Autodesk Inventor part; units mm, degrees
ref_plane "YZ Plane" through (0, 0, 0) normal (1, 0, 0) x (0, 1, 0)
ref_plane "XZ Plane" through (0, 0, 0) normal (0, 1, 0) x (-1, 0, 0)
ref_plane "XY Plane" through (0, 0, 0) normal (0, 0, 1) x (1, 0, 0)
sketch "Sketch1" plane through (0, 0, 0) normal (0, 0, 1) x (1, 0, 0)
  line L0 (-11.8, 0) -> (-11.8, 3)
  line L1 (-11.8, 3) -> (-5.8, 3)
  line L2 (-5.8, 3) -> (-5.8, 11)
  line L3 (-5.8, 11) -> (-1.4, 11)
  line L4 (-1.4, 11) -> (-1.4, 3)
  line L5 (-1.4, 3) -> (1.4, 3)
  line L6 (1.4, 3) -> (1.4, 11)
  line L7 (1.4, 11) -> (5.8, 11)
  line L8 (5.8, 11) -> (5.8, 3)
  line L9 (5.8, 3) -> (11.8, 3)
  line L10 (11.8, 3) -> (11.8, 0)
  line L11 (11.8, 0) -> (-11.8, 0)
  point P0 (0, 0)
  dimension "d0" = 3
  dimension "d1" = 6
  dimension "d2" = 8
  dimension "d3" = 4.4
  dimension "d4" = 2.8
  dimension "d5" = 4.4
  dimension "d6" = 6
  dimension "d7" = 1.4
  dimension "d8" = 0
extrude "Extrusion1" add sketch "Sketch1" along normal blind 6.5
sketch "Sketch2" plane through (-11.8, 0, 0) normal (0, -1, 0) x (1, 0, 0)
  circle A0 centre (2.8, 3.25) radius 1.5
  circle A1 centre (20.8, 3.25) radius 1.5
  line L0 (23.6, 0) -> (23.6, 6.5)
  line L1 (0, 0) -> (0, 6.5)
  line L2 (23.6, 0) -> (0, 0)
  line L3 (0, 6.5) -> (23.6, 6.5)
  line L4 (11.8, 17.7341) -> (11.8, -9.1991) construction
  line L5 (10.4, 0) -> (10.4, 6.5) construction
  line L6 (13.2, 0) -> (13.2, 6.5) construction
  point P0 (11.8, 0)
  dimension "d11" = 3
  dimension "d12" = 3
  dimension "d13" = 18
  dimension "d14" = 23.6
  dimension "d15" = 2.8
  dimension "d16" = 6.5
  dimension "d17" = 3.25
  dimension "d18" = 3.25
  dimension "d34" = 2.8
  dimension "d35" = 1.4
extrude "Extrusion2" cut sketch "Sketch2" against normal through all contours A0 | A1
sketch "Sketch3" plane through (-11.8, 0, 0) normal (0, -1, 0) x (1, 0, 0)
  line L0 (-9.1, 8.25) -> (23.9, 8.25)
  line L1 (23.9, 8.25) -> (23.9, -1.75)
  line L2 (23.9, -1.75) -> (-9.1, -1.75)
  line L3 (-9.1, -1.75) -> (-9.1, 8.25)
  line L4 (23.6, 0) -> (23.6, 6.5)
  line L5 (23.6, 0) -> (0, 0)
  line L6 (0, 6.5) -> (23.6, 6.5)
  circle A0 centre (2.8, 3.25) radius 1.5
  circle A1 centre (20.8, 3.25) radius 1.5
  point P0 (11.8, 0)
  dimension "d21" = 10
  dimension "d22" = 33
  dimension "d23" = 0.3
  dimension "d24" = 6.5
  dimension "d25" = 1.75
extrude "Extrusion3" add sketch "Sketch3" along normal blind 2
sketch "Sketch4" plane through (-11.8, -2, 0) normal (0, -1, 0) x (1, 0, 0)
  line L0 (-8.8, 8.25) -> (-2.8, 8.25)
  line L1 (-2.8, 8.25) -> (-2.8, -1.75)
  line L2 (-2.8, -1.75) -> (-8.8, -1.75)
  line L3 (-8.8, -1.75) -> (-8.8, 8.25)
  line L4 (-9.1, -1.75) -> (23.9, -1.75)
  line L5 (-9.1, -1.75) -> (-9.1, 8.25)
  point P0 (11.8, 0)
  dimension "d28" = 10
  dimension "d29" = 6
  dimension "d30" = 0
  dimension "d31" = 0.3
extrude "Extrusion4" add sketch "Sketch4" along normal blind 10
equation "\"d15\" = -0.5 * d13 + 0.5 * d14"
equation "\"d17\" = 0.5 * d16"
equation "\"d18\" = d17"
equation "\"d25\" = -0.5 * d24 + 0.5 * d21"
properties part number "optical endstop"
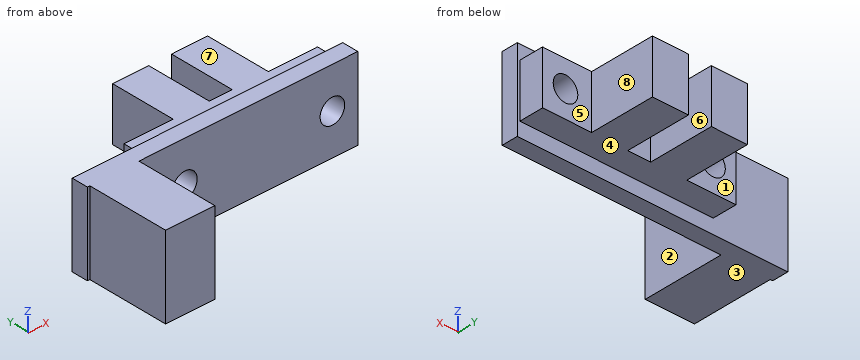
The listing builds one solid part. Answer for the finished solid, in the listing's coordinates (mm). Face numbers are marked on the shaded views. A direction names the side the tool comes from. Give positions to 0.01 mm unless a question says otherwise; leave off trailing zeros. Order: outer loops, then holes, each group sorted by start corner. A loop starts at its lowest first (then second) coordinate and runs counter-clockwise, first axis right, second up. Notation, with made-up numbers: (80, -8.5) - (106, -8.5) arc R19 cw to (106, 16.5) - close; hole circle Ø1 at (1.5, 73). An arc over 180 degrees is marked (long way). Use one line per item in the form item = value. Start each with the question number.
(1) The mould has two halves that part along X. Classify the marked faces 6, 7 and 8: released by +X, released by -X, zero draft, split by the parting line, or undercut.
(2) A cutting plane is placed at B-B, the plane y = 9.5. Write down the section's boundary in (x, z), then the cut area to 3 significant figures.
(3) A cutting plane is placed at D-D, the plane y = 1.25. Write down the section's boundary in (x, z).
(4) A cutting plane is placed at A-A, the plane x = 9. Write down the section's boundary in (y, z), then the cut area to 3 significant figures.
(5) A cutting plane is placed at C-C, the plane z = 4. Write down the section's boundary in (x, y).
(6) Flat-ended cylindrical pins translate along their axes: pin 1 Ø3.5 at (x, z) = (9, 3.25) entering from +Y; pin 2 Ø5 at (y, z) = (8.5, 4.5) entering from -X; pin 3 Ø12 at (x, y) = (2, 6.5) entering from +Z. Find the tip coordinate at first contact, or state that the pin passes through.
(7) Consider line 1 (X direction, y = 3.25, z = 0.5); line 2 (Z direction, x = -9, y = -0.35); line 3 (X direction, y = -0.25, z = 2.75). Determine where each line is inside the solid, lowest interval first. Write a range as from..to.
(8) For the marked faces 1, 2, 3, 4 and 5, determine the directions among +Z, -Z, +X, -X, +Y, -Y from which every point of the face is accessible in a straight line to the end or side of a thin tool.
Ans:
q1.face_6 = undercut
q1.face_7 = zero draft
q1.face_8 = released by +X
q2.outline = (-5.8, 0) - (-1.4, 0) - (-1.4, 6.5) - (-5.8, 6.5) - close; (1.4, 0) - (5.8, 0) - (5.8, 6.5) - (1.4, 6.5) - close
q2.area = 57.2 mm^2
q3.outline = (-11.8, 0) - (11.8, 0) - (11.8, 6.5) - (-11.8, 6.5) - close; hole circle Ø3 at (-9, 3.25); hole circle Ø3 at (9, 3.25)
q4.outline = (-2, -1.75) - (0, -1.75) - (0, 0) - (3, 0) - (3, 1.75) - (-2, 1.75) - close; (-2, 4.75) - (3, 4.75) - (3, 6.5) - (0, 6.5) - (0, 8.25) - (-2, 8.25) - close
q4.area = 24.5 mm^2
q5.outline = (-20.9, -2) - (-20.6, -2) - (-20.6, -12) - (-14.6, -12) - (-14.6, -2) - (-10.3, -2) - (-10.3, 3) - (-11.8, 3) - (-11.8, 0) - (-20.9, 0) - close; (-7.7, -2) - (7.7, -2) - (7.7, 3) - (5.8, 3) - (5.8, 11) - (1.4, 11) - (1.4, 3) - (-1.4, 3) - (-1.4, 11) - (-5.8, 11) - (-5.8, 3) - (-7.7, 3) - close; (10.3, -2) - (12.1, -2) - (12.1, 0) - (11.8, 0) - (11.8, 3) - (10.3, 3) - close
q6.pin_1 = 3
q6.pin_2 = -5.8
q6.pin_3 = 6.5
q7.line_1 = -5.8..-1.4, 1.4..5.8
q7.line_2 = -1.75..1.75, 4.75..8.25
q7.line_3 = -20.9..-10.41, -7.59..7.59, 10.41..12.1
q8.face_1 = +Z, -Z, -X, +Y
q8.face_2 = +Z, -Z, +X, -Y
q8.face_3 = -Z, +X, -X, +Y, -Y
q8.face_4 = -Z, +X, -X, +Y
q8.face_5 = +Z, -Z, +X, +Y
